from build123d import *

# Parameters (mm, degrees)
SKETCH_W        = 57
SKETCH_H        = 92
PAD_DEPTH       = 2
SKETCH001_W     = 57
SKETCH001_H     = 92
SKETCH001_W_2   = 53
SKETCH001_H_2   = 88
PAD001_DEPTH    = 17
SKETCH002_R     = 2.35
SKETCH002_R_2   = 1.35
SKETCH002_R_3   = 2
PAD002_DEPTH    = 6
SKETCH003_W     = 55
SKETCH003_H     = 90
POCKET_DEPTH    = 2
SKETCH004_W     = 13.1
SKETCH004_H     = 10.7
POCKET001_DEPTH = 1.4
SKETCH005_R     = 1.4
PAD003_DEPTH    = 1.6
SKETCH006_W     = 4
SKETCH006_H     = 4
POCKET002_DEPTH = 0.6
SKETCH007_W     = 11
SKETCH007_H     = 6
POCKET003_DEPTH = 2
SKETCH008_R     = 2
POCKET004_DEPTH = 5


with BuildPart() as part:
    # Sketch → Pad (new body)
    with BuildSketch(Plane.XY):
        Rectangle(SKETCH_W, SKETCH_H)
    extrude(amount=-PAD_DEPTH)

    # Sketch001 (on Face5 of Pad) → Pad001 (join)
    with BuildSketch(Plane.XY):
        Rectangle(SKETCH001_W, SKETCH001_H)
        Rectangle(SKETCH001_W_2, SKETCH001_H_2, mode=Mode.SUBTRACT)
    extrude(amount=PAD001_DEPTH)

    # Sketch002 (on Face15 of Pad001) → Pad002 (join)
    with BuildSketch(Plane.XY):
        with Locations((-20.841524, 32.145128)):
            Circle(SKETCH002_R)
        with Locations((-20.841524, 32.145128)):
            Circle(SKETCH002_R_2, mode=Mode.SUBTRACT)
        with Locations((20.158476, 32.145128)):
            Circle(SKETCH002_R)
        with Locations((20.158476, 32.145128)):
            Circle(SKETCH002_R_2, mode=Mode.SUBTRACT)
        with Locations((20.158476, -32.054872)):
            Circle(SKETCH002_R_3)
        with Locations((20.158476, -32.054872)):
            Circle(SKETCH002_R_2, mode=Mode.SUBTRACT)
        with Locations((-20.841524, -32.054872)):
            Circle(SKETCH002_R)
        with Locations((-20.841524, -32.054872)):
            Circle(SKETCH002_R_2, mode=Mode.SUBTRACT)
    extrude(amount=PAD002_DEPTH)

    # Sketch003 (on Face9 of Pad002) → Pocket (cut)
    with BuildSketch(Plane.XY.offset(17)):
        Rectangle(SKETCH003_W, SKETCH003_H)
    extrude(amount=-POCKET_DEPTH, mode=Mode.SUBTRACT)

    # Sketch004 (on Face16 of Pocket) → Pocket001 (cut)
    with BuildSketch(Plane.XZ.offset(-44)):
        with Locations((11.95, 6.95)):
            Rectangle(SKETCH004_W, SKETCH004_H)
    extrude(amount=-POCKET001_DEPTH, mode=Mode.SUBTRACT)

    # Sketch005 (on Face29 of Pocket001) → Pad003 (join)
    with BuildSketch(Plane.XZ.offset(-45.4)):
        with Locations((15.6, 4.5)):
            Circle(SKETCH005_R)
    extrude(amount=PAD003_DEPTH)

    # Sketch006 (on Face29 of Pad003) → Pocket002 (cut)
    with BuildSketch(Plane.XZ.offset(-45.4)):
        with Locations((14, 9.1)):
            Rectangle(SKETCH006_W, SKETCH006_H)
    extrude(amount=-POCKET002_DEPTH, mode=Mode.SUBTRACT)

    # Sketch007 (on Face8 of Pad003) → Pocket003 (cut)
    with BuildSketch(Plane.YZ.offset(28.5)):
        with Locations((4.5, 14)):
            Rectangle(SKETCH007_W, SKETCH007_H)
    extrude(amount=-POCKET003_DEPTH, mode=Mode.SUBTRACT)

    # Sketch008 (on Face14 of Pocket003) → Pocket004 (cut)
    with BuildSketch(Plane.XZ.offset(46)):
        with Locations((6.5, 12)):
            Circle(SKETCH008_R)
        with Locations((11.5, 12)):
            Circle(SKETCH008_R)
        with Locations((16.5, 12)):
            Circle(SKETCH008_R)
        with Locations((1.5, 12)):
            Circle(SKETCH008_R)
    extrude(amount=-POCKET004_DEPTH, mode=Mode.SUBTRACT)


solid = part.part
CAD build for the part. Positions are in the model's coordinates, mm. A direction names the side the tool comes from. Round coordinates to 2 decimals unless told otherwise and drop trailing zeros. Loops run counter-clockwise (first coordinate to the right, second up) from the corner with the lowest first, then second, coordinate; pieces in that order, holes last.
(1) Drop flat-ended pins along their axis: pin 1 (2 mm diameter, centred on x = 20, y = 32, fed in from +Z); pin 2 (12 mm diameter, centred on x = 19.5, y = 26, fed in from +Z); pin 3 (5 mm diameter, centred on x = 15, z = 12, fed in from -Y). Give the stop position or say it passes through.
(2) Cut at D-D (y = 3.5). Give the cut face in (x, z).
(3) Two-plate mould, pull along X, no slides. Class faces 4 (the flat face through (28.5, -1, 7)), 5 (the flat face through (0, 1, -2)), 6 (the flat face through (20.1, 30.6, 6)): +X half, -X half, draft (parallel to the pull), parting line (faces both ways), or undercut.
(4) Wall check: line 1 along X through (y, z) = (19.5, 12.25); line 2 along Y through (x, z) = (-4.5, 11.5); line 3 along Y through (x, z) = (10.5, 7.25). Give the ranges that are in metal, low to high.
(5) Which spindle directions (+Z, -Z, +X, -X, +Y, -Y) get a long thin tool onto all of the face, cutting with end or side? Do faces 1 (the cylindrical face through (10.026, -45.014, 13.352)), 2 (the flat face through (-21, -32, 0)), 3 (the flat face through (28, 10, 13)). Say none if no direction does.
(6) Cut at A-A (x = 6.5). Give the cut face in (y, z).
(7) Cut at C-C (x = -5.5). Give the cut face in (y, z), plus the area to 3 significant figures.
(8) Cut at B-B (z = 4.5). State how many separate pieces and enclosed holes the cut face has, plus the area to 3 significant figures.
Findings below:
1. pin 1: stops at z = 0
1. pin 2: stops at z = 6
1. pin 3: stops at y = -46
2. outline: (-28.5, -2) - (28.5, -2) - (28.5, 11) - (26.5, 11) - (26.5, 0) - (-26.5, 0) - (-26.5, 15) - (-27.5, 15) - (-27.5, 17) - (-28.5, 17) - close
3. face 4: +X half
3. face 5: draft
3. face 6: undercut
4. line 1: x = -28.5 to -26.5, 26.5 to 28.5
4. line 2: y = -46 to -44, 44 to 46
4. line 3: y = -46 to -44, 45.4 to 46
5. face 1: -Y
5. face 2: +Z
5. face 3: +Z, +X
6. outline: (-46, -2) - (46, -2) - (46, 17) - (45, 17) - (45, 15) - (44, 15) - (44, 12.3) - (45.4, 12.3) - (45.4, 1.6) - (44, 1.6) - (44, 0) - (-44, 0) - (-44, 10) - (-46, 10) - close; (-46, 14) - (-44, 14) - (-44, 15) - (-45, 15) - (-45, 17) - (-46, 17) - close
7. outline: (-46, -2) - (46, -2) - (46, 17) - (45, 17) - (45, 15) - (44, 15) - (44, 0) - (-44, 0) - (-44, 15) - (-45, 15) - (-45, 17) - (-46, 17) - close
7. area: 248 mm2
8. separate pieces: 5
8. enclosed holes: 5
8. area: 608 mm2
